Design review of the part shown in the three views and the two pictorial views. Dimensions are in mm from the part's minimum x, y and z. Round coordinates to 2 decimals unless told otherwise and drop trailing zeros. Order: outer loops, then holes, each group sorted by start corner. A loop starts at its lowest first (then second) coordinate and runs counter-clockwise, first axis right, second up.
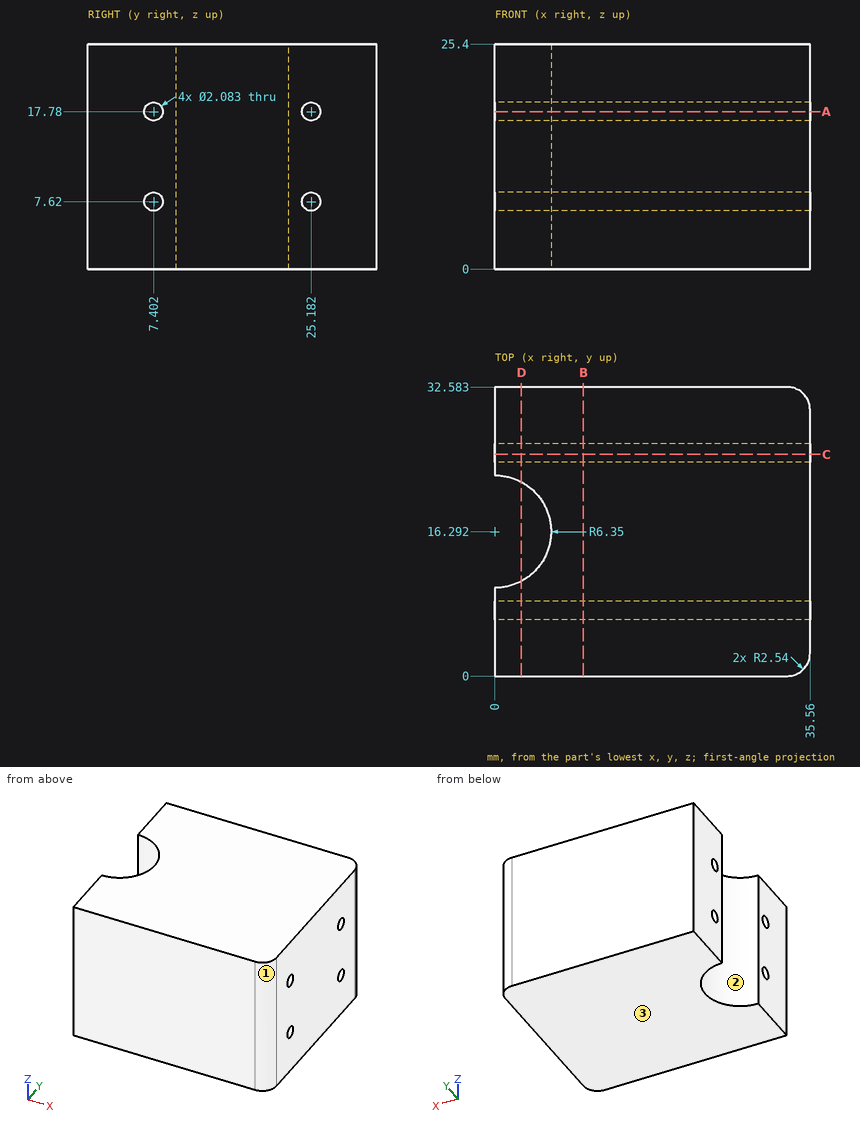
(1) Add section D-D on x = 3. Give the boundary of the cut face in (y, z) (1 decimal), plus the area to 3 significant figures.
(2) Wall thickness on L1, parallel to Z at x = 31, y = 26 (1 decimal); L2, parallel to Y at x = 22.5, z = 17.25 (1 decimal); L3, parallel to Y at x = 21, z = 8.25 (1 decimal): over which ranges is each line inside the solid? List them lowest first.
(3) Add section B-B on x = 10. Give the boundary of the cut face in (y, z), plus the area to 3 significant figures.
(4) Draft analysis for pull direction Y (two halves, no side actions). For the marked faces 1, 2 and 3, state which applies: pulls with the +Y half, pulls with the -Y half, needs draft (parallel to the pull), parting line crosses it, or undercut.
(5) Clearance check with flat-ended pins moving along their axes: P1, Ø4, axis at y = 20, z = 21, coming from the -X side; P2, Ø10, axis at x = 31.5, y = 21, coming from the -Z side. State where each tip first meets the part, or that it passes through.
(6) Add section C-C on y = 25. Give the boundary of the cut face in (x, z) (1 decimal).
(7) Add section A-A on z = 17.78. Give the boundary of the cut face in (x, y).
Here are the results:
1. outline: (0, 0) - (10.7, 0) - (10.7, 25.4) - (0, 25.4) - close; (21.9, 0) - (32.6, 0) - (32.6, 25.4) - (21.9, 25.4) - close; hole circle Ø2.1 at (7.4, 7.6); hole circle Ø2.1 at (7.4, 17.8); hole circle Ø2.1 at (25.2, 7.6); hole circle Ø2.1 at (25.2, 17.8)
1. area: 530 mm2
2. L1: z = 0 to 7, 8.3 to 17.1, 18.4 to 25.4
2. L2: y = 0 to 6.5, 8.3 to 24.3, 26.1 to 32.6
2. L3: y = 0 to 6.6, 8.2 to 24.4, 26 to 32.6
3. outline: (0, 0) - (32.58, 0) - (32.58, 25.4) - (0, 25.4) - close; hole circle Ø2.08 at (7.4, 7.62); hole circle Ø2.08 at (7.4, 17.78); hole circle Ø2.08 at (25.18, 7.62); hole circle Ø2.08 at (25.18, 17.78)
3. area: 814 mm2
4. face 1: pulls with the -Y half
4. face 2: undercut
4. face 3: needs draft
5. P1: stops at x = 2.78
5. P2: stops at z = 0
6. outline: (0, 0) - (35.6, 0) - (35.6, 6.6) - (0, 6.6) - close; (0, 8.6) - (35.6, 8.6) - (35.6, 16.8) - (0, 16.8) - close; (0, 18.8) - (35.6, 18.8) - (35.6, 25.4) - (0, 25.4) - close
7. outline: (0, 0) - (33.02, 0) arc R2.54 ccw to (35.56, 2.54) - (35.56, 6.36) - (0, 6.36) - close; (0, 8.44) - (35.56, 8.44) - (35.56, 24.14) - (0, 24.14) - (0, 22.64) arc R6.35 cw to (0, 9.94) - close; (0, 26.22) - (35.56, 26.22) - (35.56, 30.04) arc R2.54 ccw to (33.02, 32.58) - (0, 32.58) - close
